Part model, mm, in its own coordinate system. A direction names the side the tool comes from. Coordinates: 2 decimals unless noted, no trailing zeros. Write each loop counter-clockwise with the first axis right and the second up, starting at its lowest first coordinate (ties: lowest second). Pieces come first, ordered by that corner, then holes. Notation, with made-up numbers: (76, -22) - (120, -22) arc R23 cw to (120, -1) - close; hole circle Ø11 at (88, 20.25). An arc over 180 degrees is marked (long way). Use a Markdown table: item, result.
Autodesk Inventor part; units mm, degrees
ref_plane "YZ Plane" through (0, 0, 0) normal (1, 0, 0) x (0, 1, 0)
ref_plane "XZ Plane" through (0, 0, 0) normal (0, 1, 0) x (-1, 0, 0)
ref_plane "XY Plane" through (0, 0, 0) normal (0, 0, 1) x (1, 0, 0)
sketch "Sketch1" plane through (0, 0, 0) normal (0, 0, 1) x (1, 0, 0)
  line L0 (-69.85, -50.8) -> (69.85, -50.8) construction
  line L1 (69.85, -50.8) -> (69.85, 50.8) construction
  line L2 (69.85, 50.8) -> (-69.85, 50.8) construction
  line L3 (-69.85, 50.8) -> (-69.85, -50.8) construction
  line L4 (-69.85, -50.8) -> (69.85, 50.8) construction
  line L5 (69.85, -50.8) -> (-69.85, 50.8) construction
  circle A0 centre (-25.4, 57.15) radius 25.4 construction
  circle A1 centre (50.8, -12.7) radius 14.2875 construction
  circle A2 centre (50.8, -12.7) radius 19.05 construction
  line L6 (-69.85, 31.9409) -> (2.9726, -19.05) construction
  line L7 (2.9726, -19.05) -> (2.9726, -50.8) construction
  line L8 (29.21, -50.8) -> (29.21, -41.91) construction
  line L9 (29.21, -41.91) -> (50.8, -38.1) construction
  line L10 (50.8, -38.1) -> (50.8, -31.75) construction
  line L11 (69.85, -12.7) -> (64.2945, 50.8) construction
  line L12 (2.9726, -50.8) -> (29.21, -50.8)
  line L13 (29.21, -50.8) -> (29.21, -41.91)
  line L14 (50.8, -38.1) -> (50.8, -31.75)
  line L15 (69.85, -12.7) -> (64.2945, 50.8)
  line L16 (64.2945, 50.8) -> (-0.8066, 50.8)
  line L17 (-69.85, 50.8) -> (-49.9934, 50.8)
  line L18 (-69.85, 50.8) -> (-69.85, 31.9409)
  line L19 (-69.85, 31.9409) -> (2.9726, -19.05)
  line L20 (2.9726, -19.05) -> (2.9726, -50.8)
  circle A3 centre (50.8, -12.7) radius 14.2875
  arc A4 (-49.9934, 50.8) -> (-0.8066, 50.8) centre (-25.4, 57.15) ccw
  circle A5 centre (50.8, -38.1) radius 3.81
  arc A6 (50.8, -31.75) -> (69.85, -12.7) centre (50.8, -12.7) ccw
  line L21 (50.8, -38.1) -> (50.8, -44.4954)
  line L22 (50.8, -44.4954) -> (29.21, -41.91)
  circle A7 centre (24.4475, -41.275) radius 4.7625 construction
  point P0 (0, 0)
  point P1 (50.8, -34.29)
  point P2 (50.8, -41.91)
  dimension "d0" = 101.6
  dimension "d1" = 139.7
  dimension "d3" = 50.8
  dimension "d4" = 6.35
  dimension "d6" = 19.05
  dimension "d7" = 38.1
  dimension "d8" = 38.1
  dimension "d9" = 28.575
  dimension "d10" = 125
  dimension "d11" = 31.75
  dimension "d12" = 88.9
  dimension "d15" = 8.89
  dimension "d18" = 95
  dimension "d25" = 7.62
  dimension "d26" = 25.4
  dimension "d28" = 4.7625
  dimension "d31" = 6.35
  dimension "d33" = 21.59
  dimension "d38" = 76.2
  dimension "d40" = 9.525
  dimension "d49" = 9.525
extrude "Extrusion1" add sketch "Sketch1" along normal blind 6.35 contours L20 L19 L18 L17 A4 L16 L15 A6 L14 A5 L21 L22 L13 L12
fillet "Fillet1" radius 3.175 8 edges at (29.21, -50.8, 3.175) (29.21, -41.91, 3.175) (64.2945, 50.8, 3.175) (-0.8066, 50.8, 3.175) (-49.9934, 50.8, 3.175) (-69.85, 50.8, 3.175) (-69.85, 31.9409, 3.175) (2.9726, -19.05, 3.175)
chamfer "Chamfer1" distance 22.225 angle 45 1 edges at (2.9726, -50.8, 3.175)
fillet "Fillet3" radius 3.175 2 edges at (2.9726, -28.575, 3.175) (25.1976, -50.8, 3.175)
fillet "Fillet4" radius 3.175 4 edges at (50.8, -31.75, 3.175) (50.8, -34.29, 3.175) (50.8, -41.91, 3.175) (50.8, -44.4954, 3.175)
hole "Hole1" at (50.8, -12.7, 0) at (24.4475, -41.275, 0) direction (0, 0, 1) diameter 5.1054 end through all
properties part number "CL1-002" material "Aluminum 6061"
Item 1: Band-saw the part on A-A, the plane x = 15. Give the cut face in (y, z).
From the geometry:
| item | result |
|---|---|
| outline | (-40.6, 0) - (50.8, 0) - (50.8, 6.35) - (-40.6, 6.35) - close |
Item 2: Two-plate mould, pull along Y, no slides. Class faces 4 (the face through (-33.93, 6.79, 3.13)), 5 (the face through (15, 12, 6.35)), 6 (the face through (47.703, 1.248, 3.131)), 7 (the face through (50.32, -42.64, 3.13)): pulls with the +Y half, pulls with the -Y half, needs draft (parallel to the pull), parting line crosses it, or undercut.
From the geometry:
| item | result |
|---|---|
| face 4 | pulls with the -Y half |
| face 5 | needs draft |
| face 6 | undercut |
| face 7 | undercut |
Item 3: Band-saw the part on B-B, the plane z = 1. Count the separate pieces of the cut face and the enclosed holes in it, then the cut area to 3 significant figures.
From the geometry:
| item | result |
|---|---|
| separate pieces | 1 |
| enclosed holes | 2 |
| area | 7,610 mm^2 |
Item 4: Drill centre lines: probe 1 along X at (y, z) = (43, 4.25); probe 2 along X at (y, z) = (-16, 0.75); probe 3 along Y at (x, z) = (56.5, 0.5). Where is each one in solid material? Low to high.
From the geometry:
| item | result |
|---|---|
| probe 1 | -69.85 to -46.49, -4.31 to 64.98 |
| probe 2 | -1.38 to 36.9, 64.7 to 69.56 |
| probe 3 | -30.88 to -25.8, 0.4 to 50.8 |
Item 5: Which spindle directions (+Z, -Z, +X, -X, +Y, -Y) get a long thin tool onto all of the face, cutting with end or side? Do faces 1 (the face through (-50.485, 50.201, 3.219)), 2 (the face through (41.378, -43.367, 3.131)), 3 (the face through (2.973, -24, 3)). Say none if no direction does.
From the geometry:
| item | result |
|---|---|
| face 1 | +Z, -Z, +Y |
| face 2 | +Z, -Z, -Y |
| face 3 | +Z, -Z, -X, -Y |
Item 6: Drop flat-ended pins along their axis: P1, Ø2, axis at x = -28, z = 2.5, coming from the -Y side; P2, Ø3, axis at y = -24, z = 3, coming from the -X side; P3, Ø1.3, axis at y = -46, z = 3, coming from the +X side. Give the stop position or say it passes through.
From the geometry:
| item | result |
|---|---|
| P1 | y = 1.94 |
| P2 | x = 2.97 |
| P3 | x = 29.21 |
Item 7: Band-saw the part on C-C, the plane y = 22. Give the cut face in (x, z).
From the geometry:
| item | result |
|---|---|
| outline | (-55.65, 0) - (66.81, 0) - (66.81, 6.35) - (-55.65, 6.35) - close |
